Source: CAD feature listing. Evaluate the final solid. Frame: model axes, mm. A direction names the side the tool comes from. Give positions to 0.01 mm unless a question says otherwise; leave off trailing zeros. Order: outer loops, then holes, each group sorted by start corner. A loop starts at its lowest first (then second) coordinate and runs counter-clockwise, first axis right, second up. Notation, with made-up numbers: (74, -32.75) -> (107, -32.75) arc R8 cw to (107, -18.75) -> close; hole circle Ø11 at (46, 17). An arc over 180 degrees is marked (long way). Use CSV: the item, a comma, the result in double quotes.
```python
from build123d import *

# Parameters (mm, degrees)
SKETCH1_W                    = 34
SKETCH1_H                    = 3
BASE_FLANGE1_DEPTH           = 50
EDGE_FLANGE1_STRIP_W         = 13.4732
EDGE_FLANGE1_STRIP_H         = 3
EDGE_FLANGE1_STRIP_CUT_DEPTH = 34
EDGE_FLANGE1_DEPTH           = 34
SKETCH9_R                    = 3
CUT_EXTRUDE1_DEPTH           = 10
SKETCH10_R                   = 3
CUT_EXTRUDE2_DEPTH           = 10


# Sheet-metal steps are written as plain solids
with BuildPart() as part:
    # Sketch1 → Base-Flange1 (new body)
    with BuildSketch(Plane(origin=(0, 0, 0), x_dir=(1, 0, 0), z_dir=(0, 1, 0))):
        with Locations((17, -1.5)):
            Rectangle(SKETCH1_W, SKETCH1_H)
    extrude(amount=BASE_FLANGE1_DEPTH)

    # Edge-Flange1 strip (across the edge) → Edge-Flange1 strip cut (cut)
    with BuildSketch(Plane(origin=(34, 50, 3), x_dir=(0, -1, 0), z_dir=(-1, 0, 0))):
        with Locations((-3, -1.5)):
            Rectangle(EDGE_FLANGE1_STRIP_W, EDGE_FLANGE1_STRIP_H)
    extrude(amount=EDGE_FLANGE1_STRIP_CUT_DEPTH, mode=Mode.SUBTRACT)

    # Edge-Flange1 section (across the edge) → Edge-Flange1 (add)
    with BuildSketch(Plane(origin=(34, 50, 3), x_dir=(0, -1, 0), z_dir=(-1, 0, 0))):
        with BuildLine():
            Line((0, 0.7366), (0, 77))
            Line((0, 77), (3, 77))
            Line((3, 77), (3, 0.7366))
            ThreePointArc((3, 0.7366), (3.215745145, 0.215745145), (3.7366, 0))
            Line((3.7366, 0), (3.7366, -3))
            ThreePointArc((3.7366, -3), (1.094424801, -1.905575199), (0, 0.7366))
        make_face()
    extrude(amount=EDGE_FLANGE1_DEPTH)

    # Sketch9 → Cut-Extrude1 (cut)
    with BuildSketch(Plane(origin=(0, 50, 0), x_dir=(1, 0, 0), z_dir=(0, 1, 0))):
        with Locations(Location((17, -70.19, 0), (0, 0, 270))):
            Circle(SKETCH9_R)
    extrude(amount=-CUT_EXTRUDE1_DEPTH, mode=Mode.SUBTRACT)

    # Sketch10 → Cut-Extrude2 (cut)
    with BuildSketch(Plane.XY.offset(3)):
        with Locations((17, 23.1317)):
            Circle(SKETCH10_R)
    extrude(amount=-CUT_EXTRUDE2_DEPTH, mode=Mode.SUBTRACT)


solid = part.part
```
1. Mould query, pull axis Z, two halves, no side actions, for faces 3 (the cylindrical face through (17.24, 48.88, 1.07)), 4 (the cylindrical face through (15.175, 48.521, 67.809)), 5 (the flat face through (17, 0, 1)). Classes: released by +Z, released by -Z, zero draft, split by the parting line, or undercut.
Answer below:
face 3,"released by -Z"
face 4,"undercut"
face 5,"zero draft"
2. Pin query (flat end, axial travel): P1, Ø10, axis at x = 14.5, z = 56.5, coming from the -Y side; P2, Ø10, axis at x = 11, y = 28, coming from the +Z side. Return the tip coordinate at first contact, or that it passes through.
Answer below:
P1,"stops at y = 47"
P2,"stops at z = 3"
3. Ray query, line 1 along Z through (x, y) = (9, 22); line 2 along Y through (x, z) = (30, 53); line 3 along Y through (x, z) = (17, 1.25). Return the intervals inside material, ascending.
Answer below:
line 1,"z = 0 to 3"
line 2,"y = 47 to 50"
line 3,"y = 0 to 20.13, 26.13 to 49.05"
4. Section query A-A on x = 17. Return loops of the section in (y, z), plus the area to 3 significant figures.
Answer below:
outline,"(0, 0) -> (20.13, 0) -> (20.13, 3) -> (0, 3) -> close; (26.13, 0) -> (46.26, 0) arc R3.74 ccw to (50, 3.74) -> (50, 67.19) -> (47, 67.19) -> (47, 3.74) arc R0.74 cw to (46.26, 3) -> (26.13, 3) -> close; (47, 73.19) -> (50, 73.19) -> (50, 80) -> (47, 80) -> close"
area,"342 mm²"
5. Section query B-B on z = 70.19. Return loops of the section in (x, y), plus the area to 3 significant figures.
Answer below:
outline,"(0, 47) -> (14, 47) -> (14, 50) -> (0, 50) -> close; (20, 47) -> (34, 47) -> (34, 50) -> (20, 50) -> close"
area,"84.0 mm²"
6. Access query for faces 1 (the cylindrical face through (14.619, 21.306, 1.521)), 2 (the flat face through (17, 47, 42)). Directions: +Z, -Z, +X, -X, +Y, -Y. A direction counts if a zero-diameter tool reaches every point of the face in a straight line with its end or side. Return the directions, or none.
Answer below:
face 1,"+Z, -Z"
face 2,"+Z, +X, -X, -Y"
7. Section query D-D on y = 18.5. Return loops of the section in (x, z).
Answer below:
outline,"(0, 0) -> (34, 0) -> (34, 3) -> (0, 3) -> close"
8. Section query C-C on x = 27. Return loops of the section in (y, z).
Answer below:
outline,"(0, 0) -> (46.26, 0) arc R3.74 ccw to (50, 3.74) -> (50, 80) -> (47, 80) -> (47, 3.74) arc R0.74 cw to (46.26, 3) -> (0, 3) -> close"
